The drawing under review shows one solid part. Ordinate dimensions are in mm from its lowest x, y, z. A direction names the side the tool comes from. Coordinates: 2 decimals unless noted, no trailing zeros. Write each loop counter-clockwise with the first axis right and the second up, starting at its lowest first coordinate (ties: lowest second). Pieces come first, ordered by that corner, then holes. Notation, with made-up numbers: (71.25, 55.5) - (119.25, 55.5) arc R26 ccw to (119.25, 82.5) - close; hole circle Ø5 at (32, -13.5). An arc over 180 degrees is marked (long way). Put each result on its own line as item: value. Start each with the question number.
Item 1: For pin 1 (6 mm diameter, centred on y = 12, z = 7.5, fed in from +X); pin 2 (2 mm diameter, centred on x = 28.5, z = 4, fed in from +Y); pin 3 (1.2 mm diameter, centred on x = 29.5, z = 4, fed in from -Y), all flat-tipped, find the tip position at first contact; note any pin that passes through.
Item 2: Consider section D-D on z = 3.5. Give the boundary of the cut face in (x, y).
Item 3: Consider section B-B on x = 10. Give the boundary of the cut face in (y, z).
Item 4: Consider section A-A on z = 6. Give the boundary of the cut face in (x, y).
Item 5: To check wall thickness, follow L1, parallel to Y at x = 3.5, z = 7; L2, parallel to Y at x = 21.5, z = 8.5; L3, parallel to X at y = 23, z = 3.5. State the ranges of each line that lie inside material, in increasing order. Write a range as [from, to].
Item 6: Consider section C-C on y = 5.5. Give the boundary of the cut face in (x, z), then the cut area to 3 significant figures.
Item 7: Mouldability with a two-part tool opening along X and no side actions: class the marked faces 4, 5, 6 and 7 as pulls with the +X half, pulls with the -X half, needs draft (parallel to the pull), parting line crosses it, or undercut.
Item 8: Machinability: for the marked faces 1, 2 and 3, which of the approach directions +Z, -Z, +X, -X, +Y, -Y give a long, thin tool a straight path to every point of the face, cutting with its end or side? Answer none if there is none.
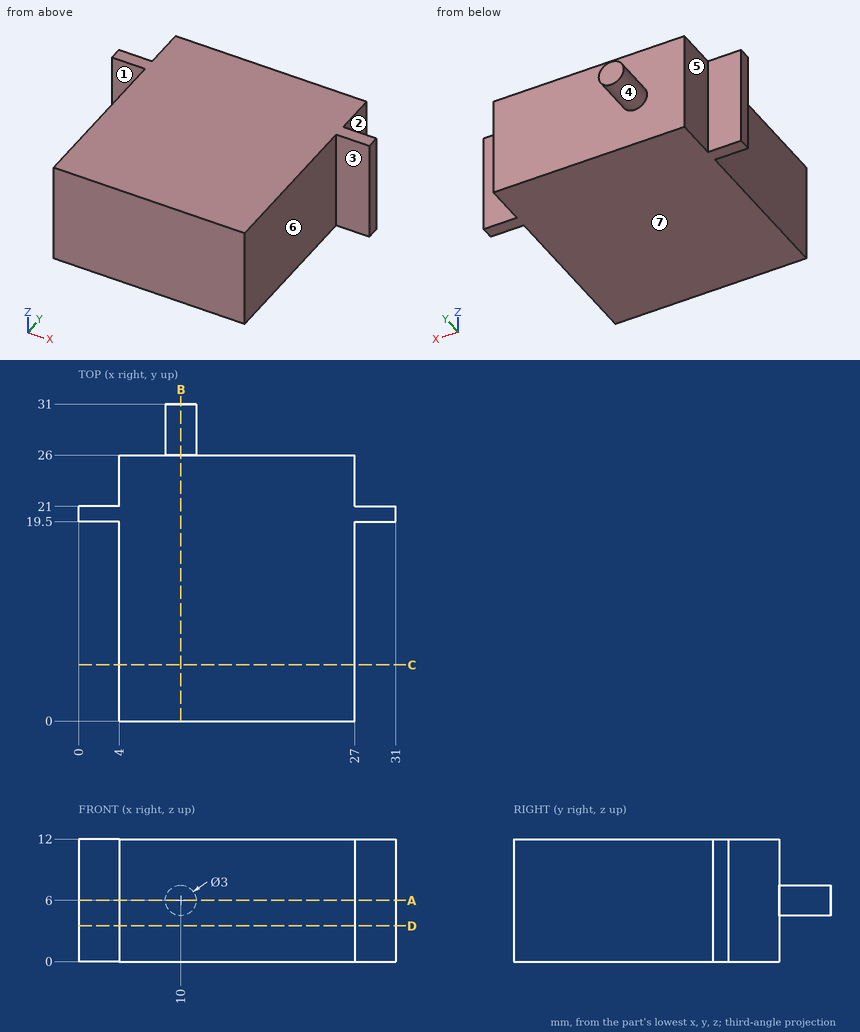
Report:
1. pin 1: x = 27
1. pin 2: y = 21
1. pin 3: y = 19.5
2. outline: (0, 19.5) - (4, 19.5) - (4, 0) - (27, 0) - (27, 19.5) - (31, 19.5) - (31, 21) - (27, 21) - (27, 26) - (4, 26) - (4, 21) - (0, 21) - close
3. outline: (0, 0) - (26, 0) - (26, 4.5) - (31, 4.5) - (31, 7.5) - (26, 7.5) - (26, 12) - (0, 12) - close
4. outline: (0, 19.5) - (4, 19.5) - (4, 0) - (27, 0) - (27, 19.5) - (31, 19.5) - (31, 21) - (27, 21) - (27, 26) - (11.5, 26) - (11.5, 31) - (8.5, 31) - (8.5, 26) - (4, 26) - (4, 21) - (0, 21) - close
5. L1: [19.5, 21]
5. L2: [0, 26]
5. L3: [4, 27]
6. outline: (4, 0) - (27, 0) - (27, 12) - (4, 12) - close
6. area: 276 mm²
7. face 4: parting line crosses it
7. face 5: pulls with the -X half
7. face 6: pulls with the +X half
7. face 7: needs draft
8. face 1: +Z, -Z, -X, -Y
8. face 2: +Z, -Z, +X, +Y
8. face 3: +Z, -Z, +X, -Y
